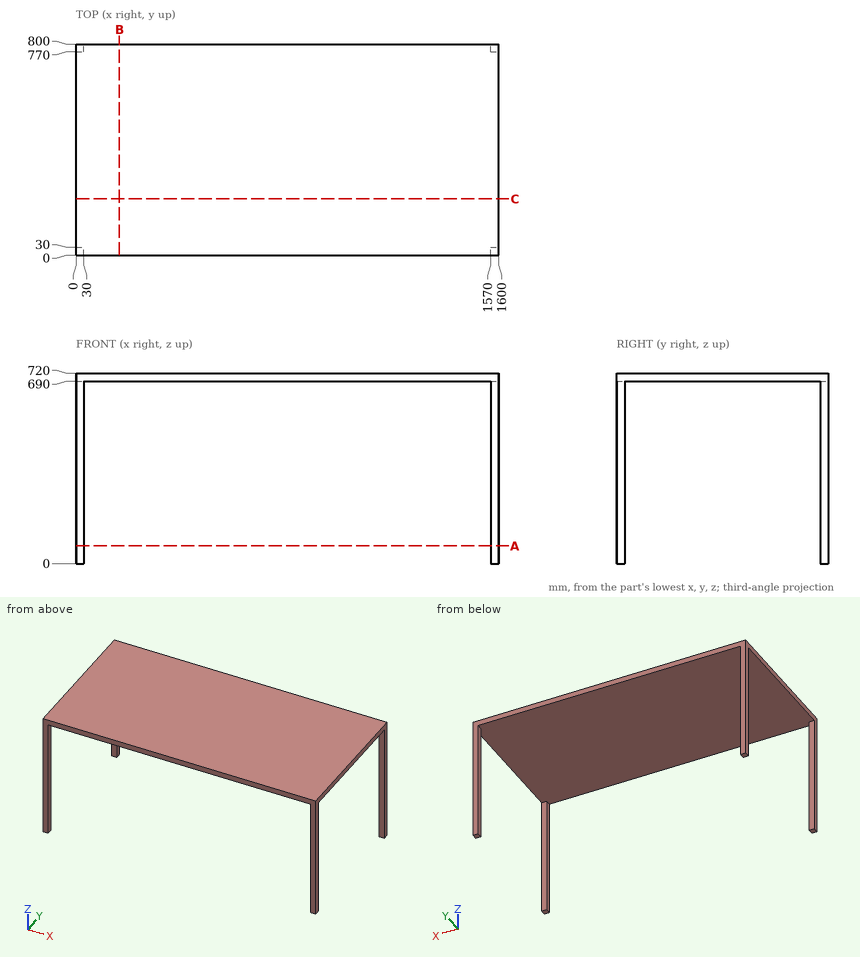
Input: dimensioned drawing with shaded views. Units: mm. Origin: part minimum x, y, z. Give positions to 0.01 mm unless a question says otherwise; leave off trailing zeros. Loops run counter-clockwise (first coordinate to the right, second up) from the corner with the lowest first, then second, coordinate; pieces in that order, holes last. Notation, with made-up numbers: (42, 30) -> (95, 30) arc R9 ccw to (95, 39) -> close; hole circle Ø1 at (0.25, 33). An arc over 180 degrees is marked (long way). Return JSON: item names as keys, results as strings.
Item 1: Section A-A, the plane z = 66.5. Output: boundary loops of the cut face in (x, y).
Filled in:
{"outline": "(0, 0) -> (30, 0) -> (30, 30) -> (0, 30) -> close; (0, 770) -> (30, 770) -> (30, 800) -> (0, 800) -> close; (1570, 0) -> (1600, 0) -> (1600, 30) -> (1570, 30) -> close; (1570, 770) -> (1600, 770) -> (1600, 800) -> (1570, 800) -> close"}
Item 2: Section B-B, the plane x = 164. Output: boundary loops of the cut face in (y, z), plus the area to 3 significant figures.
Filled in:
{"outline": "(0, 690) -> (800, 690) -> (800, 720) -> (0, 720) -> close", "area": "24,000 mm^2"}
Item 3: Line query: line 1 (Z direction, x = 1210, y = 501.5). Output: solid intervals per line, ascending.
Filled in:
{"line 1": "690 to 720"}
Item 4: Pin query (flat end, axial travel): P1, Ø5, axis at x = 420.5, y = 182.5, coming from the -Z side. Return the tip coordinate at first contact, or that it passes through.
Filled in:
{"P1": "z = 690"}
Item 5: Section C-C, the plane y = 214. Output: boundary loops of the cut face in (x, z), plus the area to 3 significant figures.
Filled in:
{"outline": "(0, 690) -> (1600, 690) -> (1600, 720) -> (0, 720) -> close", "area": "48,000 mm^2"}
